For this review, take the finished solid that the model builds, in its own axes (mm). Give positions to 0.01 mm unless a question says otherwise; leave off trailing zeros. Order: outer loops, then holes, each group sorted by start corner. A loop starts at its lowest first (then second) coordinate and runs counter-clockwise, first axis right, second up. Notation, with made-up numbers: (59, 34.25) - (102, 34.25) arc R19 cw to (102, 41.25) - close; hole circle Ø1 at (47, -15). An arc over 180 degrees is marked (long way). Answer as a JSON object with one key per item and string values. Group by question number.
from build123d import *

# Parameters (mm, degrees)
F0_W     = 120
F0_H     = 120
F0_W_2   = 4.2
F0_H_2   = 20.2
F0_W_3   = 20.2
F0_H_3   = 4.2
F1_DEPTH = 4


with BuildPart() as f1:
    # F0 (on Top) → F1 (new body)
    with BuildSketch(Plane.XY):
        Rectangle(F0_W, F0_H)
        with Locations((-52.2, 0)):
            Rectangle(F0_W_2, F0_H_2, mode=Mode.SUBTRACT)
        with Locations((52.2, 0)):
            Rectangle(F0_W_2, F0_H_2, mode=Mode.SUBTRACT)
        with Locations((0, 48.2)):
            Rectangle(F0_W_3, F0_H_3, mode=Mode.SUBTRACT)
    extrude(amount=F1_DEPTH)


solid = f1.part
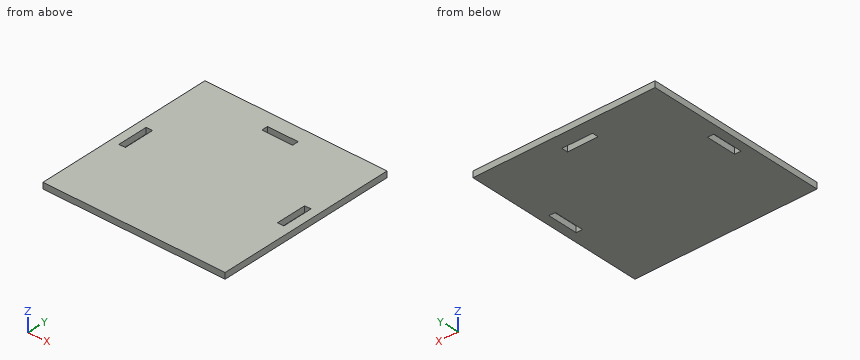
1) Consider section D-D (z = 2.2). Give the boundary of the cut face in (x, y), plus the area to 3 significant figures.
2) For line 1 (X direction, y = -9.5, z = 3.7); line 2 (Y direction, x = 53, z = 3.75), list the stretches that pass through material, from the lowest coordinate up.
3) Consider section B-B (x = 52.5). Give the boundary of the cut face in (y, z).
4) Consider section A-A (y = 4.5). Give the boundary of the cut face in (x, z).
Result set:
{
 "1": {"outline": "(-60, -60) - (60, -60) - (60, 60) - (-60, 60) - close; hole (-54.3, -10.1) - (-50.1, -10.1) - (-50.1, 10.1) - (-54.3, 10.1) - close; hole (-10.1, 46.1) - (10.1, 46.1) - (10.1, 50.3) - (-10.1, 50.3) - close; hole (50.1, -10.1) - (54.3, -10.1) - (54.3, 10.1) - (50.1, 10.1) - close", "area": "14,100 mm2"},
 "2": {"line 1": "x = -60 to -54.3, -50.1 to 50.1, 54.3 to 60", "line 2": "y = -60 to -10.1, 10.1 to 60"},
 "3": {"outline": "(-60, 0) - (-10.1, 0) - (-10.1, 4) - (-60, 4) - close; (10.1, 0) - (60, 0) - (60, 4) - (10.1, 4) - close"},
 "4": {"outline": "(-60, 0) - (-54.3, 0) - (-54.3, 4) - (-60, 4) - close; (-50.1, 0) - (50.1, 0) - (50.1, 4) - (-50.1, 4) - close; (54.3, 0) - (60, 0) - (60, 4) - (54.3, 4) - close"}
}
